```python
from build123d import *

# Parameters (mm, degrees)
BOSS_EXTRUDE1_DEPTH          = 25
BOSS_EXTRUDE2_DEPTH          = 3
M4X0_7_TAPPED_HOLE1_D        = 3.3
M4X0_7_TAPPED_HOLE1_DEPTH    = 14
M4X0_7_TAPPED_HOLE1_TIP      = 0.991420021
F_2_0_2_DIAMETER_HOLE1_D     = 2
F_2_0_2_DIAMETER_HOLE1_DEPTH = 3.512823811
F_2_0_2_DIAMETER_HOLE2_D     = 2
F_2_0_2_DIAMETER_HOLE2_DEPTH = 3.512823811
M3X0_5_TAPPED_HOLE1_D        = 2.5
M3X0_5_TAPPED_HOLE1_DEPTH    = 2


with BuildPart() as part:
    # Sketch1 → Boss-Extrude1 (new body)
    with BuildSketch(Plane.XY):
        Polygon((13.697937079, 25.419129705), (16.197937079, 25.419129705), (16.197937079, 22.619129705), (24.397937079, 22.619129705), (24.397937079, 25.419129705), (55.197937079, 25.419129705), (55.197937079, 22.619129705), (63.397937079, 22.619129705), (63.397937079, 25.419129705), (64.147937079, 25.419129705), (64.147937079, 19.106305894), (55.197937079, 19.106305894), (55.197937079, -3.66605846), (52.811898109, -6.05209743), (50.912403173, -6.05209743), (50.447937079, -5.587631336), (53.983470985, -2.05209743), (29.289533755, 22.6418398), (25.753999849, 19.106305894), (13.697937079, 19.106305894), align=None)
    extrude(amount=BOSS_EXTRUDE1_DEPTH)

    # Sketch2 → Boss-Extrude2 (add)
    with BuildSketch(Plane(origin=(0, 0, 0), x_dir=(-1, 0, 0), z_dir=(0, 0, -1))):
        Polygon((-64.147937079, 25.419129705), (-63.397937079, 25.419129705), (-63.397937079, 22.619129705), (-55.197937079, 22.619129705), (-55.197937079, 25.419129705), (-24.397937079, 25.419129705), (-24.397937079, 22.619129705), (-16.197937079, 22.619129705), (-16.197937079, 25.419129705), (-13.697937079, 25.419129705), (-13.697937079, 19.106305894), (-25.753999849, 19.106305894), (-29.289533755, 22.6418398), (-32.825067661, 19.106305894), (-29.289533755, 15.570771988), (-46.912403173, -2.05209743), (-50.447937079, 1.483436476), (-53.983470985, -2.05209743), (-50.447937079, -5.587631336), (-50.912403173, -6.05209743), (-52.811898109, -6.05209743), (-55.197937079, -3.66605846), (-55.197937079, 19.106305894), (-64.147937079, 19.106305894), align=None)
    extrude(amount=BOSS_EXTRUDE2_DEPTH)

    # M4x0.7 Tapped Hole1
    with Locations(Plane(origin=(0, 0, -3), x_dir=(-1, 0, 0), z_dir=(0, 0, -1))):
        with Locations((-46.197937079, 15.419129705)):
            Hole(M4X0_7_TAPPED_HOLE1_D / 2, depth=M4X0_7_TAPPED_HOLE1_DEPTH)
            with Locations((0, 0, -(M4X0_7_TAPPED_HOLE1_DEPTH + M4X0_7_TAPPED_HOLE1_TIP / 2))):  # 118° drill point
                Cone(0, M4X0_7_TAPPED_HOLE1_D / 2, M4X0_7_TAPPED_HOLE1_TIP, mode=Mode.SUBTRACT)

    # Ø2.0 (2) Diameter Hole1
    with Locations(Plane(origin=(0, 19.106305894, 0), x_dir=(-1, 0, 0), z_dir=(0, -1, 0))):
        with Locations((-59.297937079, -22), (-59.297937079, -16.5), (-59.297937079, -5.5), (-59.297937079, 0)):
            Hole(F_2_0_2_DIAMETER_HOLE1_D / 2, depth=F_2_0_2_DIAMETER_HOLE1_DEPTH)

    # Ø2.0 (2) Diameter Hole2
    with Locations(Plane(origin=(0, 19.106305894, 0), x_dir=(-1, 0, 0), z_dir=(0, -1, 0))):
        with Locations((-20.297937079, -22), (-20.297937079, -16.5), (-20.297937079, -5.5), (-20.297937079, 0)):
            Hole(F_2_0_2_DIAMETER_HOLE2_D / 2, depth=F_2_0_2_DIAMETER_HOLE2_DEPTH)

    # M3x0.5 Tapped Hole1
    with Locations(Plane(origin=(29.43199777, -29.43199777, 0), x_dir=(0, 0, -1), z_dir=(0.707106781, -0.707106781, 0))):
        with Locations((-11, 34.764172148)):
            Hole(M3X0_5_TAPPED_HOLE1_D / 2, depth=M3X0_5_TAPPED_HOLE1_DEPTH)


solid = part.part
```
The listing builds one solid part. Answer for the finished solid, in the listing's coordinates (mm). A direction names the side the tool comes from. Round coordinates to 2 decimals unless told otherwise and drop trailing zeros. Loops run counter-clockwise (first coordinate to the right, second up) from the corner with the lowest first, then second, coordinate; pieces in that order, holes last.
Q1. Section D-D, the plane z = 13.5 is taken. Determine the outline of the cut face in (x, y), then the cut area to 3 significant figures.
Q2. Section B-B, the plane y = 20 is taken. Count the separate pieces of the cut face and the enclosed holes in it, then the cut area to 3 significant figures.
Q3. Given pin 1 Ø4 at (y, z) = (15.5, 3) entering from -X; pin 2 Ø2.5 at (x, z) = (20.3, 16.5) entering from +Y; pin 3 Ø1.5 at (x, z) = (35, 17.5) entering from -Y; pin 4 Ø1.2 at (x, z) = (20.3, 0) entering from -Y, each flat-ended and moving along its own axis, determine where each tip first touches the part or whether it passes through.
Q4. For a pull along X with two mould halves and no side action, classify faces 4 (the face through (13.698, 22, 11)), 5 (the face through (55.049, -3.815, 11.196)), 6 (the face through (55.198, 24, 11)), 7 (the face through (46.425, 15.245, 11.819)) as released by +X, released by -X, zero draft, split by the parting line, or undercut.
Q5. Which of the six approach directions +Z, -Z, +X, -X, +Y, -Y give full straight-line access (tool end or side, diameter ignored) to faces 1 (the face through (44.55, 15.49, 4.1)), 2 (the face through (59, 22.619, 11)), 3 (the face through (31.08, 17.36, -1.48))?
Q6. Section A-A, the plane z = 22 is taken. Determine the outline of the cut face in (x, y), then the cut area to 3 significant figures.
Q7. Find the intervals of material crossed by line 1 (X direction, y = 20.95, z = 16.5); line 2 (Z direction, x = 39, y = 12); line 3 (X direction, y = 21.65, z = 22), in increasing order.
Completed:
1. outline: (13.7, 19.11) - (25.75, 19.11) - (29.29, 22.64) - (53.98, -2.05) - (50.45, -5.59) - (50.91, -6.05) - (52.81, -6.05) - (55.2, -3.67) - (55.2, 19.11) - (64.15, 19.11) - (64.15, 25.42) - (63.4, 25.42) - (63.4, 22.62) - (55.2, 22.62) - (55.2, 25.42) - (24.4, 25.42) - (24.4, 22.62) - (16.2, 22.62) - (16.2, 25.42) - (13.7, 25.42) - close
1. area: 519 mm2
2. separate pieces: 2
2. enclosed holes: 8
2. area: 1,240 mm2
3. pin 1: stops at x = 34.43
3. pin 2: stops at y = 22.62
3. pin 3: stops at y = 16.18
3. pin 4: passes through
4. face 4: released by -X
4. face 5: released by +X
4. face 6: undercut
4. face 7: undercut
5. face 1: -Z
5. face 2: +Z, -Z, +Y
5. face 3: +Z, -Z, -X
6. outline: (13.7, 19.11) - (19.3, 19.11) - (19.3, 22.62) - (16.2, 22.62) - (16.2, 25.42) - (13.7, 25.42) - close; (21.3, 19.11) - (25.75, 19.11) - (29.29, 22.64) - (53.98, -2.05) - (50.45, -5.59) - (50.91, -6.05) - (52.81, -6.05) - (55.2, -3.67) - (55.2, 19.11) - (58.3, 19.11) - (58.3, 22.62) - (55.2, 22.62) - (55.2, 25.42) - (24.4, 25.42) - (24.4, 22.62) - (21.3, 22.62) - close; (60.3, 19.11) - (64.15, 19.11) - (64.15, 25.42) - (63.4, 25.42) - (63.4, 22.62) - (60.3, 22.62) - close
6. area: 505 mm2
7. line 1: x = 13.7 to 19.3, 21.3 to 27.6, 30.98 to 58.3, 60.3 to 64.15
7. line 2: z = -3 to 0
7. line 3: x = 13.7 to 19.3, 21.3 to 28.3, 30.28 to 58.3, 60.3 to 64.15
